from build123d import *

# Parameters (mm, degrees)
F0_W     = 110
F0_H     = 110
F1_DEPTH = 2
F2_W     = 10
F2_H     = 10
F3_DEPTH = 50
F4_W     = 80
F4_H     = 80
F5_DEPTH = 52.001


with BuildPart() as f1:
    # F0 (on Top) → F1 (new body)
    with BuildSketch(Plane.XY):
        Rectangle(F0_W, F0_H)
    extrude(amount=-F1_DEPTH)

    # F2 (on face) → F3 (join)
    with BuildSketch(Plane(origin=(0, 0, -2), x_dir=(1, 0, 0), z_dir=(0, 0, -1))):
        with Locations((-50, -50)):
            Rectangle(F2_W, F2_H)
        with Locations((-50, 50)):
            Rectangle(F2_W, F2_H)
        with Locations((50, 50)):
            Rectangle(F2_W, F2_H)
        with Locations((50, -50)):
            Rectangle(F2_W, F2_H)
    extrude(amount=F3_DEPTH)

    # F4 (on face) → F5 (cut, through all)
    with BuildSketch(Plane.XY):
        Rectangle(F4_W, F4_H)
    extrude(amount=-F5_DEPTH, mode=Mode.SUBTRACT)


solid = f1.part
For this review, take the finished solid that the model builds, in its own axes (mm). A direction names the side the tool comes from. Coordinates: 2 decimals unless noted, no trailing zeros. Order: outer loops, then holes, each group sorted by start corner. A loop starts at its lowest first (then second) coordinate and runs counter-clockwise, first axis right, second up. Notation, with made-up numbers: (0, 21) -> (42, 21) arc R26 cw to (42, 36) -> close; hole circle Ø9 at (-22.75, 84). An arc over 180 degrees is marked (long way). Return JSON: item names as keys, results as strings.
1. We need section A-A on y = 28. Write out the cut boundary in (x, z).
Answer block:
{"outline": "(-55, -2) -> (-40, -2) -> (-40, 0) -> (-55, 0) -> close; (40, -2) -> (55, -2) -> (55, 0) -> (40, 0) -> close"}
2. For line 1 (Y direction, x = -46.5, z = -32.5); line 2 (Z direction, x = 5.5, y = 46.5), list the stretches that pass through material, from the lowest coordinate up. Write a range as from..to.
Answer block:
{"line 1": "-55..-45, 45..55", "line 2": "-2..0"}
3. The part is to be moulded in two halves that separate along X. For faces 1 (the flat face through (55, -8, -1)), 2 (the flat face through (45, 50, -27)), 3 (the flat face through (50, 45, -27)), say which applies: +X half, -X half, draft (parallel to the pull), parting line (faces both ways), or undercut.
Answer block:
{"face 1": "+X half", "face 2": "undercut", "face 3": "draft"}
4. We need section D-D on y = 42. Write out the cut boundary in (x, z), and give its area (3 significant figures).
Answer block:
{"outline": "(-55, -2) -> (55, -2) -> (55, 0) -> (-55, 0) -> close", "area": "220 mm²"}
5. We need section B-B on z = -29.5. Write out the cut boundary in (x, y), and give its area (3 significant figures).
Answer block:
{"outline": "(-55, -55) -> (-45, -55) -> (-45, -45) -> (-55, -45) -> close; (-55, 45) -> (-45, 45) -> (-45, 55) -> (-55, 55) -> close; (45, -55) -> (55, -55) -> (55, -45) -> (45, -45) -> close; (45, 45) -> (55, 45) -> (55, 55) -> (45, 55) -> close", "area": "400 mm²"}
6. For pin 1 Ø12 at (y, z) = (38, -12.5) entering from -X, flat-tipped, find the tip position at first contact; note if it passes through.
Answer block:
{"pin 1": "through"}
7. Machinability: for faces 4 (the flat face through (-50, 45, -27)), 5 (the flat face through (50, 50, -52)), 6 (the flat face through (-45, 50, -27)), which of the approach directions +Z, -Z, +X, -X, +Y, -Y give a long, thin tool a straight path to every point of the face, cutting with its end or side? Answer none if there is none.
Answer block:
{"face 4": "-Z, +X, -X", "face 5": "-Z, +X, -X, +Y, -Y", "face 6": "-Z, +Y, -Y"}
